Design review of the part built by this model. Coordinates are the model's own, in mm. A direction names the side the tool comes from. Give positions to 0.01 mm unless a question says otherwise; leave off trailing zeros. Loops run counter-clockwise (first coordinate to the right, second up) from the corner with the lowest first, then second, coordinate; pieces in that order, holes last. Notation, with made-up numbers: (83.5, 58) - (123.5, 58) arc R21 cw to (123.5, 97) - close; hole circle Ø10 at (62.25, 32.25). An arc over 180 degrees is marked (long way). Write each question's results on one line, items separated by ' | '.
from build123d import *

# Parameters (mm, degrees)
SKETCH1_R           = 28
BOSS_EXTRUDE1_DEPTH = 7
BOSS_EXTRUDE2_START = -1.226475693
SKETCH4_R           = 5
BOSS_EXTRUDE2_DEPTH = 6.232399738


with BuildPart() as part:
    # Sketch1 → Boss-Extrude1 (new body)
    with BuildSketch(Plane(origin=(0, 0, 0), x_dir=(1, 0, 0), z_dir=(0, 1, 0))):
        with Locations(Location((0, 0, 0), (0, 0, 270))):
            Circle(SKETCH1_R)
    extrude(amount=BOSS_EXTRUDE1_DEPTH)

    # Sketch4 → Boss-Extrude2 (add)
    with BuildSketch(Plane.XY.offset(22).offset(BOSS_EXTRUDE2_START)):
        with BuildLine():
            Line((-6.241476895, 15.467624234), (-6.241476895, 7))
            ThreePointArc((-6.241476895, 7), (0, 5.970563029), (6.241476895, 7))
            Line((6.241476895, 7), (6.241476895, 15.467624234))
            Line((6.241476895, 15.467624234), (6.241476895, 23.956480862))
            ThreePointArc((6.241476895, 23.956480862), (0, 30.197957757), (-6.241476895, 23.956480862))
            Line((-6.241476895, 23.956480862), (-6.241476895, 15.467624234))
        make_face()
        with Locations((0, 23.956480862)):
            Circle(SKETCH4_R, mode=Mode.SUBTRACT)
    boss_extrude2 = extrude(amount=BOSS_EXTRUDE2_DEPTH)

    # Mirror1: Boss-Extrude2 across plane
    add(boss_extrude2.mirror(Plane.XY))


solid = part.part
(1) Insertion check: P1, Ø9, axis at x = 0, y = 23.96, coming from the +Z side; P2, Ø3, axis at y = 18, z = 22.5, coming from the -X side; P3, Ø7, axis at y = 14, z = -23.5, coming from the +X side; P4, Ø17, axis at x = -5, z = -9.5, coming from the +Y side. Each pin has a flat end and moves straight along its axis. Give the tip position at first contact, or say it passes through.
Answers below:
P1: through | P2: x = -6.24 | P3: x = 6.24 | P4: y = 7
(2) Take a section at D-D on x = -14. Give the boundary of the cut face in (y, z), plus the area to 3 significant figures.
Answers below:
outline: (0, -24.25) - (7, -24.25) - (7, 24.25) - (0, 24.25) - close | area: 339 mm2
(3) Take a section at A-A on x = 0. Give the boundary of the cut face in (y, z), plus the area to 3 significant figures.
Answers below:
outline: (0, -28) - (7, -28) - (7, -27.01) - (18.96, -27.01) - (18.96, -20.77) - (7, -20.77) - (7, 20.77) - (18.96, 20.77) - (18.96, 27.01) - (7, 27.01) - (7, 28) - (0, 28) - close; (28.96, -27.01) - (30.2, -27.01) - (30.2, -20.77) - (28.96, -20.77) - close; (28.96, 20.77) - (30.2, 20.77) - (30.2, 27.01) - (28.96, 27.01) - close | area: 557 mm2
(4) Wall thickness on line 1 along Y through (x, z) = (0, 25); line 2 along Z through (x, y) = (-2, 17); line 3 along Y through (x, z) = (-14.5, -10.5): over which ranges is each line inside the solid? List them lowest first. Write a range as from..to.
Answers below:
line 1: 0..18.96, 28.96..30.2 | line 2: -27.01..-20.77, 20.77..27.01 | line 3: 0..7
(5) Take a section at B-B on z = 23. Give the boundary of the cut face in (x, y), plus the area to 3 significant figures.
Answers below:
outline: (-15.97, 0) - (15.97, 0) - (15.97, 7) - (6.24, 7) - (6.24, 23.96) arc R6.24 ccw to (-6.24, 23.96) - (-6.24, 7) - (-15.97, 7) - close; hole circle Ø10 at (0, 23.96) | area: 418 mm2
(6) Take a section at C-C on z = 0. Give the boundary of the cut face in (x, y).
Answers below:
outline: (-28, 0) - (28, 0) - (28, 7) - (-28, 7) - close
(7) Tool access review of faces 5 (the flat face through (0, 16, -27.006)), 6 (the flat face through (-6.241, 16, 24)), 7 (the flat face through (0, 16, 27.006)), 8 (the flat face through (6.241, 15, -24)), 9 (the flat face through (0, 16, 20.774)): name each direction out of +Z, -Z, +X, -X, +Y, -Y from which nothing blocks a thin tool from reaching the whole face with its end or side.
Answers below:
face 5: -Z, +X, -X, +Y | face 6: +Z, -Z, -X, +Y | face 7: +Z, +X, -X, +Y | face 8: +Z, -Z, +X, +Y | face 9: +X, -X, +Y
(8) Draft analysis for pull direction X (two halves, no side actions). For faces 1 (the flat face through (0, 0, 0)), 2 (the cylindrical face through (-1.084, 19.075, -23.846)), 3 (the cylindrical face through (-1.084, 19.075, 23.846)), 4 (the cylindrical face through (-27.334, 3.451, -6.07)), state which applies: pulls with the +X half, pulls with the -X half, needs draft (parallel to the pull), parting line crosses it, or undercut.
Answers below:
face 1: needs draft | face 2: undercut | face 3: undercut | face 4: parting line crosses it
